Part model, mm, in its own coordinate system. A direction names the side the tool comes from. Coordinates: 2 decimals unless noted, no trailing zeros. Loops run counter-clockwise (first coordinate to the right, second up) from the corner with the lowest first, then second, coordinate; pieces in that order, holes last. Notation, with made-up numbers: M 5.5,39.25 L 37.5,39.25 A23 cw 37.5,64.25 Z; hole C 78.5,76 d10. An arc over 180 degrees is marked long. Answer as a JSON object with one key per item and string values. Group by question number.
1. Saw through at D-D on y = -2.75. Write the cut outline in (x, z).
2. Saw through at A-A on x = 0. Write the cut outline in (y, z).
3. Drop flat-ended pins along their axis: pin 1 Ø3 at (y, z) = (-4.5, 1) entering from +X; pin 2 Ø1 at (x, y) = (-6.5, -1.5) entering from +Z; pin 3 Ø3 at (x, y) = (0, 0) entering from +Z. Give the stop position or say it passes through.
4. Mould opens along Y. For faces 3 (the face through (0, -2, 6)), 4 (the face through (-0.867, -3.905, 4.451)), 5 (the face through (-2, -1, 8)), 6 (the face through (0, 0, 4)) say: released by +Y, released by -Y, zero draft, split by the parting line, or undercut.
5. 3-axis set-ups, long thin cutter, end or side, ignore diameter. For faces 1 (the face through (0, -5, 1)), 2 (the face through (-2.38, -10.74, 0.49)): which of +Z, -Z, +X, -X, +Y, -Y reach the whole face in a straight line?
6. Saw through at C-C on z = 5. Write the cut outline in (x, y), then the cut area to 3 significant figures.
7. Drill centre lines: L1, parallel to Y at x = 0, z = 6.85; L2, parallel to Z at x = 8.5, y = -5.75; L3, parallel to Y at x = -0.5, z = 7.5. Where is each one in solid material? Low to high.
from build123d import *

# Parameters (mm, degrees)
F0_R     = 11
F0_R_2   = 4
F1_DEPTH = 1
F2_R     = 4
F3_DEPTH = 7
F4_R     = 2
F5_DEPTH = 4


with BuildPart() as f1:
    # F0 (on Top) → F1 (new body)
    with BuildSketch(Plane.XY):
        Circle(F0_R)
        Circle(F0_R_2, mode=Mode.SUBTRACT)
        Circle(F0_R_2)
    extrude(amount=F1_DEPTH)

    # F2 (on face) → F3 (join)
    with BuildSketch(Plane.XY.offset(1)):
        Circle(F2_R)
    extrude(amount=F3_DEPTH)

    # F4 (on face) → F5 (cut)
    with BuildSketch(Plane.XY.offset(8)):
        Circle(F4_R)
    extrude(amount=-F5_DEPTH, mode=Mode.SUBTRACT)


solid = f1.part
Outcome:
{
 "1": {"outline": "M -10.65,0 L 10.65,0 L 10.65,1 L 2.9,1 L 2.9,8 L -2.9,8 L -2.9,1 L -10.65,1 Z"},
 "2": {"outline": "M -11,0 L 11,0 L 11,1 L 4,1 L 4,8 L 2,8 L 2,4 L -2,4 L -2,8 L -4,8 L -4,1 L -11,1 Z"},
 "3": {"pin 1": "stops at x = 10.58", "pin 2": "stops at z = 1", "pin 3": "stops at z = 4"},
 "4": {"face 3": "undercut", "face 4": "split by the parting line", "face 5": "zero draft", "face 6": "undercut"},
 "5": {"face 1": "+Z", "face 2": "+Z, -Z"},
 "6": {"outline": "C 0,0 d8; hole C 0,0 d4", "area": "37.7 mm²"},
 "7": {"L1": "y = -4 to -2, 2 to 4", "L2": "z = 0 to 1", "L3": "y = -3.97 to -1.94, 1.94 to 3.97"}
}
